Autodesk Inventor part; units mm, degrees
ref_plane "YZ Plane" through (0, 0, 0) normal (1, 0, 0) x (0, 1, 0)
ref_plane "XZ Plane" through (0, 0, 0) normal (0, 1, 0) x (-1, 0, 0)
ref_plane "XY Plane" through (0, 0, 0) normal (0, 0, 1) x (1, 0, 0)
sketch "Sketch1" plane through (0, 0, 0) normal (0, 0, 1) x (1, 0, 0)
  line L0 (0, 0) -> (0, 7.9375) construction
  line L1 (0, 25.4) -> (12.7, 25.4)
  line L2 (12.7, 25.4) -> (12.7, 28.575)
  line L3 (12.7, 28.575) -> (14.2875, 28.575)
  line L4 (14.2875, 28.575) -> (14.2875, 12)
  line L5 (14.2875, 12) -> (8.2875, 12)
  line L6 (8.2875, 12) -> (8.2875, 7.9375)
  line L7 (8.2875, 7.9375) -> (0, 7.9375)
  line L8 (0, 0) -> (14.2875, 0) construction
  line L9 (14.2875, 0) -> (14.2875, 12) construction
  line L10 (0, 7.9375) -> (0, 25.4)
  dimension "d3" = 25.4
  dimension "d4" = 28.575
  dimension "d5" = 12
  dimension "d6" = 7.9375
  dimension "d7" = 6
  dimension "d8" = 14.2875
  dimension "d9" = 1.5875
revolve "Revolution1" add sketch "Sketch1" angle 360 about axis through (0, 0, 0) along (1, 0, 0)
mirror "Mirror1" about plane through (0, 25.4, 0) normal (-1, 0, 0)
sketch "Sketch2" plane through (-14.2875, 0, 0) normal (-1, 0, 0) x (0, 0, 1)
  circle A0 centre (0, 0) radius 12
  circle A1 centre (0, 0) radius 28.575
  circle A2 centre (0, 0) radius 15.875 construction
  line L0 (0, 0) -> (0, 15.875) construction
  circle A3 centre (0, 15.875) radius 2.54 construction
  circle A4 centre (-13.7482, -7.9375) radius 2.54 construction
  circle A5 centre (13.7482, -7.9375) radius 2.54 construction
  circle A6 centre (0, 0) radius 20.6375
  point P0 (0, 13.335)
  point P1 (0, 12)
  dimension "d11" = 5.08
  dimension "d27" = 31.75
  dimension "d15" = 360
  dimension "d28" = 5.08
  dimension "d29" = 5.08
  dimension "d40" = 41.275
chamfer "Chamfer1" distance 0.7937 angle 45 2 edges at (-14.2875, -28.575, 0) (14.2875, -28.575, 0)
extrude "Extrusion2" add sketch "Sketch2" along normal blind 0.7937 contours A6
sketch "Sketch4" plane through (-15.0812, 0, 0) normal (-1, 0, 0) x (0, 0, 1)
  point P0 (0, 15.875)
  point P1 (-13.7482, -7.9375)
  point P2 (13.7482, -7.9375)
hole "Hole3" at (-15.0812, -7.9375, 13.7482) at (-15.0812, -7.9375, -13.7482) at (-15.0813, 15.875, 0) direction (1, 0, 0) diameter 3.302 depth 12.7 tip angle 118
properties part number "Wheel" material "Aluminum 6061"
CAD build for the part. Positions are in the model's coordinates, mm. A direction names the side the tool comes from. Coordinates: 2 decimals unless noted, no trailing zeros. Order: outer loops, then holes, each group sorted by start corner. A loop starts at its lowest first (then second) coordinate and runs counter-clockwise, first axis right, second up.
Item 1: Band-saw the part on B-B on x = 0. List the corners of the cut face in (y, z) (1 decimal).
Check sheet entries:
outline: circle Ø50.8 at (0, 0); hole circle Ø15.9 at (0, 0)
Item 2: Two-plate mould, pull along X, no slides. Class faces 4 (the face through (-8.642, -7.305, 15.273)), 5 (the face through (12.7, -26, -2)), 6 (the face through (8.288, 2, -8)), 7 (the face through (-15.081, -9, 9)): +X half, -X half, draft (parallel to the pull), parting line (faces both ways), or undercut.
Check sheet entries:
face 4: draft
face 5: undercut
face 6: +X half
face 7: -X half
Item 3: Pin check, flat tips, straight feed: pin 1 Ø1 at (x, z) = (-3, 9.5) entering from +Y; pin 2 Ø6 at (x, y) = (5, -12) entering from +Z; pin 3 Ø12 at (x, z) = (5.5, 20.5) entering from +Y; pin 4 Ø7 at (y, z) = (-1.5, -3.5) entering from -X. Stop position of each tip, or through.
Check sheet entries:
pin 1: stops at y = 23.75
pin 2: stops at z = 23.75
pin 3: stops at y = 20.85
pin 4: passes through
Item 4: 3-axis set-ups, long thin cutter, end or side, ignore diameter. For faces 1 (the face through (11.25, -11.99, -0.53)), 2 (the face through (-8.642, -6.326, -14.106)), 3 (the face through (-12.7, 26, -2)): which of +Z, -Z, +X, -X, +Y, -Y reach the whole face in a straight line?
Check sheet entries:
face 1: +X
face 2: -X
face 3: none
Item 5: Band-saw the part on D-D on x = 10.75. List the corners of the cut face in (y, z).
Check sheet entries:
outline: circle Ø50.8 at (0, 0); hole circle Ø24 at (0, 0)
Item 6: Drill centre lines: L1, parallel to Z at x = -0.75, y = 0; L2, parallel to Z at x = 10.8, y = 0; L3, parallel to X at y = 11, z = -25. Where is each one in solid material? Low to high.
Check sheet entries:
L1: z = -25.4 to -7.94, 7.94 to 25.4
L2: z = -25.4 to -12, 12 to 25.4
L3: x = -14.29 to -12.7, 12.7 to 14.29
Item 7: Band-saw the part on C-C on x = -5.25. List the corners of the cut face in (y, z) (1 decimal).
Check sheet entries:
outline: circle Ø50.8 at (0, 0); hole circle Ø3.3 at (-7.9, -13.7); hole circle Ø3.3 at (-7.9, 13.7); hole circle Ø15.9 at (0, 0); hole circle Ø3.3 at (15.9, 0)
